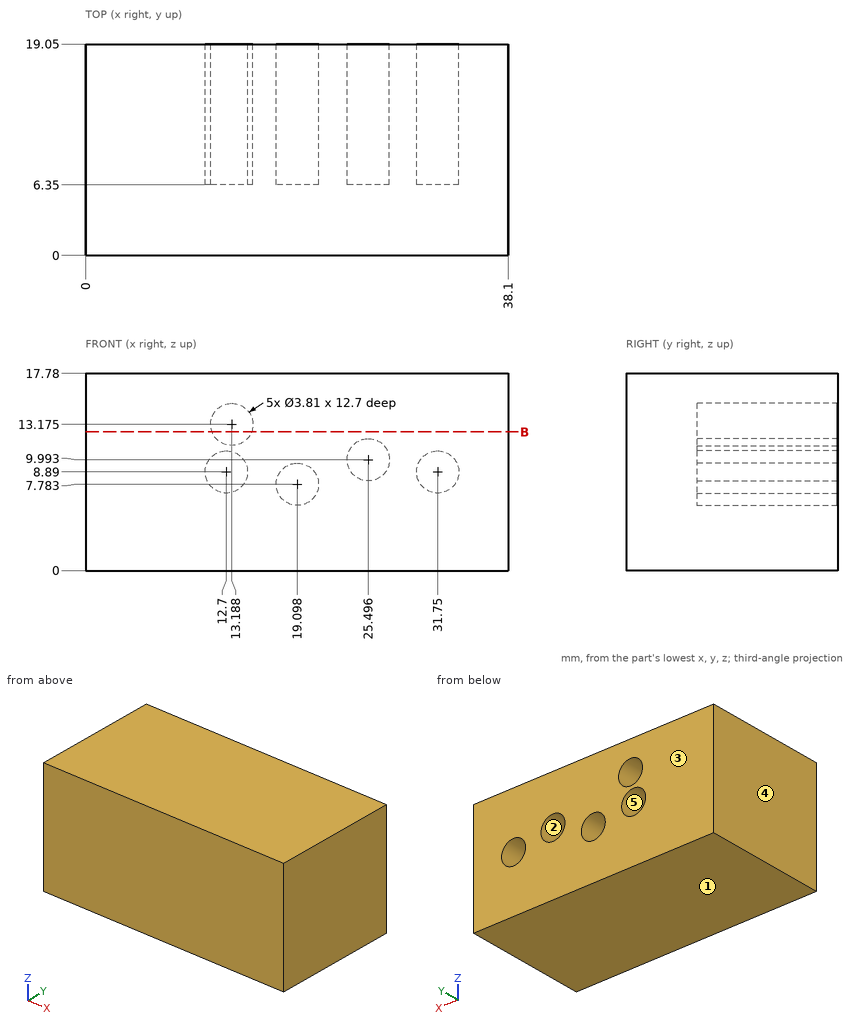
Study the drawing (mm; zero at the part's minimum x, y, z) and answer. A direction names the side the tool comes from. Round coordinates to 2 decimals unless told otherwise and drop trailing zeros. Order: outer loops, then holes, each group sorted by start corner. A loop starts at its lowest first (then second) coordinate and runs counter-clockwise, first axis right, second up. Notation, with made-up numbers: (84, -11) - (126, -11) arc R24 cw to (126, 9) - close; hole circle Ø1 at (-5, 37.25). An arc over 180 degrees is marked (long way). Use one line per item in the form item = value. Start each with the question number.
(1) Find the intervals of material crossed by line 1 along X through (y, z) = (9, 13) (1 decimal); line 2 along Z through (x, y) = (18, 9) (1 decimal); line 3 along Y through (x, z) = (11.5, 9), in increasing order. Write a range as from..to.
(2) The part is cut by section B-B (z = 12.5). Give the vertices of the cut face in (x, y).
(3) A flat-ended cylindrical pin translates along its axis: pin 1 Ø1.1 at (x, z) = (31, 9.5) entering from +Y. Find the tip coordinate at first contact, or state that the pin passes through.
(4) Determine the mould class of the marked faces 3, 4 and 5 for opening direction X: +X half, -X half, draft (parallel to the pull), parting line (faces both ways), or undercut.
(5) For the marked faces 1 and 2, determine the directions among +Z, -Z, +X, -X, +Y, -Y from which every point of the face is accessible in a straight line to the end or side of a thin tool.
Checked values:
q1.line_1 = 0..11.3, 15.1..38.1
q1.line_2 = 0..6.2, 9.3..17.8
q1.line_3 = 0..6.35
q2.outline = (0, 0) - (38.1, 0) - (38.1, 19.05) - (14.97, 19.05) - (14.97, 6.35) - (11.41, 6.35) - (11.41, 19.05) - (0, 19.05) - close
q3.pin_1 = 6.35
q4.face_3 = draft
q4.face_4 = -X half
q4.face_5 = undercut
q5.face_1 = -Z, +X, -X, +Y, -Y
q5.face_2 = +Y
